Work out the finished part from the listing and answer in its coordinate system (mm). A direction names the side the tool comes from. Coordinates: 2 decimals unless noted, no trailing zeros. Order: outer loops, then holes, each group sorted by start corner. A loop starts at its lowest first (then second) coordinate and runs counter-clockwise, first axis right, second up. Notation, with made-up numbers: (-12.5, -27.75) -> (25.5, -27.75) arc R31 ccw to (25.5, 7.25) -> close; hole circle Ø7 at (47, 4). An arc over 180 degrees is marked (long way). Use one line per item in the form item = value.
Autodesk Fusion 360 part; units mm, degrees
sketch "Sketch1" plane through (0, 0, 0) normal (0, 0, 1) x (1, 0, 0)
  line L0 (27.2658, -132.272) -> (-30, -99.2094)
  line L1 (-30, -99.2094) -> (-30, -33.0822)
  line L2 (-30, -33.0822) -> (27.2658, -0.0196)
  line L3 (27.2658, -0.0196) -> (84.5305, -33.0822)
  line L4 (84.5305, -33.0822) -> (84.5305, -99.2094)
  line L5 (84.5305, -99.2094) -> (27.2658, -132.272)
  line L6 (-8.1812, -86.62) -> (27.2658, -107.0932)
  line L7 (27.2658, -107.0932) -> (62.7117, -86.62)
  line L8 (62.7117, -86.62) -> (62.7117, -45.6716)
  line L9 (62.7117, -45.6716) -> (27.2658, -25.1985)
  line L10 (27.2658, -25.1985) -> (-8.1812, -45.6716)
  line L11 (-8.1812, -45.6716) -> (-8.1812, -86.62)
  line L12 (16.2638, -72.502) -> (16.2638, -47.2612)
  line L13 (38.2046, -59.8516) -> (38.2046, -85.0914)
  line L14 (-30, -33.0822) -> (-30, -99.2094)
  line L15 (-8.1812, -86.62) -> (-8.1812, -45.6716)
  line L16 (-8.1812, -45.6716) -> (27.2658, -25.2594)
  line L17 (27.2658, -25.2594) -> (62.7117, -45.6716)
  line L18 (62.7117, -45.6716) -> (62.7117, -45.7326)
  line L19 (84.5305, -33.0822) -> (27.2658, -0.0196)
  line L20 (27.2658, -0.0196) -> (-30, -33.0822)
  line L21 (38.2046, -59.8516) -> (38.2046, -85.0914)
  line L22 (13.6721, -99.2419) -> (-8.1812, -86.62)
  line L23 (40.8862, -33.0655) -> (62.7117, -45.7326)
  line L24 (27.2658, -25.2594) -> (62.7117, -45.7326)
  line L25 (-8.1812, -86.62) -> (27.2658, -107.0932)
  line L26 (16.2638, -47.2612) -> (40.8862, -33.0655)
  line L27 (27.2658, -25.2594) -> (-8.1812, -45.6716)
  line L28 (-8.1812, -86.62) -> (-8.1812, -45.6716)
  line L29 (-8.1812, -86.62) -> (16.3868, -72.44)
  line L30 (16.3868, -72.44) -> (16.2638, -47.2612)
  line L31 (16.2638, -47.2612) -> (40.8862, -33.0655)
  line L32 (38.2046, -85.0914) -> (13.6721, -99.2419)
  line L33 (13.6721, -99.2419) -> (27.2658, -107.0932)
  line L34 (62.7117, -86.62) -> (62.7117, -45.7326)
  line L35 (27.2658, -107.0932) -> (62.7117, -86.62)
  line L36 (38.2046, -85.0914) -> (38.2046, -59.8516)
  line L37 (38.2046, -59.8516) -> (62.7117, -45.7326)
extrude "Extrude1" add sketch "Sketch1" along normal blind 10 contours L0 L1 L2 L3 L4 L5 L14 L19 L20 | L6 L13 L21 L22 L24 L25 L26 L29 L30 L31 L32 L36 L37 makes body 1
sketch "Sketch2" plane through (0, 0, 10) normal (0, 0, 1) x (1, 0, 0)
  line L0 (62.7117, -45.6716) -> (62.7117, -45.7326)
  line L1 (62.7117, -45.7326) -> (62.7117, -86.62)
  line L2 (62.7117, -86.62) -> (27.2658, -107.0932)
  line L3 (27.2658, -107.0932) -> (13.6721, -99.2419)
  line L4 (13.6721, -99.2419) -> (38.2046, -85.0914)
  line L5 (38.2046, -85.0914) -> (38.2046, -59.8516)
  line L6 (38.2046, -59.8516) -> (62.7117, -45.7326)
  line L7 (40.8333, -33.0959) -> (16.2638, -47.2612)
  line L8 (16.2638, -47.2612) -> (16.3868, -72.44)
  line L9 (16.3868, -72.44) -> (-8.1812, -86.62)
  line L10 (-8.1812, -86.62) -> (-8.1812, -45.6716)
  line L11 (-8.1812, -45.6716) -> (27.2658, -25.1985)
  line L12 (84.5305, -33.0822) -> (27.2658, -0.0196)
  line L13 (27.2658, -0.0196) -> (-30, -33.0822)
  line L14 (-30, -33.0822) -> (-30, -99.2094)
  line L15 (-30, -99.2094) -> (27.2658, -132.272)
  line L16 (27.2658, -132.272) -> (84.5305, -99.2094)
  line L17 (84.5305, -99.2094) -> (84.5305, -33.0822)
extrude "Extrude2" add 1 faces at (3.646, -110.2411, 10) along direction (0, 0, 1) blind 7 separate body on bodies 1 makes body 2
sketch "Sketch3" plane through (0, 0, 17) normal (0, 0, 1) x (1, 0, 0)
  line L0 (62.7117, -45.6716) -> (62.7117, -45.7326)
  line L1 (62.7117, -45.7326) -> (62.7117, -86.62)
  line L2 (62.7117, -86.62) -> (27.2658, -107.0932)
  line L3 (27.2658, -107.0932) -> (13.6721, -99.2419)
  line L4 (13.6721, -99.2419) -> (38.2046, -85.0914)
  line L5 (38.2046, -85.0914) -> (38.2046, -59.8516)
  line L6 (38.2046, -59.8516) -> (62.7117, -45.7326)
  line L7 (40.8333, -33.0959) -> (16.2638, -47.2612)
  line L8 (16.2638, -47.2612) -> (16.3868, -72.44)
  line L9 (16.3868, -72.44) -> (-8.1812, -86.62)
  line L10 (-8.1812, -86.62) -> (-8.1812, -45.6716)
  line L11 (-8.1812, -45.6716) -> (27.2658, -25.1985)
  line L12 (84.5305, -33.0822) -> (27.2658, -0.0196)
  line L13 (27.2658, -0.0196) -> (-30, -33.0822)
  line L14 (-30, -33.0822) -> (-30, -99.2094)
  line L15 (-30, -99.2094) -> (27.2658, -132.272)
  line L16 (27.2658, -132.272) -> (84.5305, -99.2094)
  line L17 (84.5305, -99.2094) -> (84.5305, -33.0822)
  line L18 (-30, -33.0822) -> (27.2658, -0.0196)
  line L19 (84.5305, -33.0822) -> (27.2658, -0.0196)
  line L20 (-30, -33.0822) -> (-30, -99.2094)
  line L21 (-30, -99.2094) -> (27.2658, -132.272)
  line L22 (27.2658, -132.272) -> (84.5305, -99.2094)
  line L23 (84.5305, -33.0822) -> (84.5305, -99.2094)
  line L24 (-8.1812, -45.6716) -> (27.2658, -25.1985)
  line L25 (16.2638, -47.2612) -> (40.8333, -33.0959)
  line L26 (16.2638, -47.2612) -> (16.3868, -72.44)
  line L27 (-8.1812, -86.62) -> (16.3868, -72.44)
  line L28 (-8.1812, -86.62) -> (-8.1812, -45.6716)
  line L29 (62.7117, -45.6716) -> (38.2046, -59.8516)
  line L30 (38.2046, -85.0914) -> (13.6721, -99.2419)
  line L31 (27.2658, -107.0932) -> (13.6721, -99.2419)
  line L32 (27.2658, -107.0932) -> (62.7117, -86.62)
  line L33 (62.7117, -86.62) -> (62.7117, -45.6716)
  line L34 (38.2046, -85.0914) -> (38.2046, -59.8516)
  line L35 (27.2658, -25.1985) -> (40.8333, -33.0959)
  point P0 (27.2658, -25.1985)
extrude "Extrude3" add sketch "Sketch3" along normal blind 5 separate body makes body 3
sketch "Sketch4" plane through (0, 0, 22) normal (0, 0, 1) x (1, 0, 0)
  line L0 (62.7117, -86.62) -> (27.2658, -107.0932)
  line L1 (27.2658, -107.0932) -> (13.6721, -99.2419)
  line L2 (13.6721, -99.2419) -> (38.2046, -85.0914)
  line L3 (38.2046, -85.0914) -> (38.2046, -59.8516)
  line L4 (38.2046, -59.8516) -> (62.7117, -45.6716)
  line L5 (62.7117, -45.6716) -> (62.7117, -86.62)
  line L6 (16.3868, -72.44) -> (-8.1812, -86.62)
  line L7 (-8.1812, -86.62) -> (-8.1812, -45.6716)
  line L8 (-8.1812, -45.6716) -> (27.2658, -25.1985)
  line L9 (27.2658, -25.1985) -> (40.8333, -33.0959)
  line L10 (40.8333, -33.0959) -> (16.2638, -47.2612)
  line L11 (16.2638, -47.2612) -> (16.3868, -72.44)
  line L12 (-30, -33.0822) -> (-30, -99.2094)
  line L13 (-30, -99.2094) -> (27.2658, -132.272)
  line L14 (27.2658, -132.272) -> (84.5305, -99.2094)
  line L15 (84.5305, -99.2094) -> (84.5305, -33.0822)
  line L16 (84.5305, -33.0822) -> (27.2658, -0.0196)
  line L17 (27.2658, -0.0196) -> (-30, -33.0822)
hidden bodies 1 2
(1) Straight lines are drawn through the part: line 1 along X through (y, z) = (-68, 17.35); line 2 along Y through (x, z) = (24, 21.7); line 3 along Y through (x, z) = (16.5, 19.2). For each, find the intervals that lie inside material, in ascending order.
Data:
line_1 = -30 to -8.18, 16.37 to 38.2, 62.71 to 84.53
line_2 = -130.39 to -105.21, -93.28 to -42.8, -27.08 to -1.91
line_3 = -126.06 to -100.88, -97.61 to -47.13, -31.42 to -6.24
(2) The mould has two halves that part along X. Classify faces 3 (the flat face through (26, -65, 22)), 4 (the flat face through (9.29, -35.58, 19.46)), 5 (the flat face through (84.53, -67, 19)): released by +X, released by -X, zero draft, split by the parting line, or undercut.
Data:
face_3 = zero draft
face_4 = undercut
face_5 = released by +X
(3) Section D-D on y = -79 is taken. Write down the section's boundary in (x, z), plus the area to 3 significant figures.
Data:
outline = (-30, 17) -> (-8.18, 17) -> (-8.18, 22) -> (-30, 22) -> close; (5.02, 17) -> (38.2, 17) -> (38.2, 22) -> (5.02, 22) -> close; (62.71, 17) -> (84.53, 17) -> (84.53, 22) -> (62.71, 22) -> close
area = 384 mm²
(4) Which of the six approach directions +Z, -Z, +X, -X, +Y, -Y give full straight-line access (tool end or side, diameter ignored) to faces 1 (the flat face through (55.5, -115.97, 19.46)), 2 (the flat face through (4.275, -79.431, 19.465))?
Data:
face_1 = +Z, -Z, +X, -Y
face_2 = +Z, -Z
(5) Section B-B on x = -5 is taken. Write down the section's boundary in (y, z), plus the area to 3 significant figures.
Data:
outline = (-113.64, 17) -> (-84.78, 17) -> (-84.78, 22) -> (-113.64, 22) -> close; (-43.83, 17) -> (-18.65, 17) -> (-18.65, 22) -> (-43.83, 22) -> close
area = 270 mm²
(6) Section A-A on y = -101 is taken. Write down the section's boundary in (x, z).
Data:
outline = (-26.9, 17) -> (16.72, 17) -> (16.72, 22) -> (-26.9, 22) -> close; (37.82, 17) -> (81.43, 17) -> (81.43, 22) -> (37.82, 22) -> close
(7) Section C-C on z = 20.1 is taken. Write down the section's boundary in (x, y), plus the area to 3 significant figures.
Data:
outline = (-30, -99.21) -> (27.27, -132.27) -> (84.53, -99.21) -> (84.53, -33.08) -> (27.27, -0.02) -> (-30, -33.08) -> close; hole (-8.18, -86.62) -> (16.39, -72.44) -> (16.26, -47.26) -> (40.83, -33.1) -> (27.27, -25.2) -> (-8.18, -45.67) -> close; hole (13.67, -99.24) -> (27.27, -107.09) -> (62.71, -86.62) -> (62.71, -45.67) -> (38.2, -59.85) -> (38.2, -85.09) -> close
area = 8,800 mm²
(8) Each of these flat-tipped pins is pushed along its axis until it touches: P1, Ø1, axis at x = 37.5, z = 19, coming from the +Y side; P2, Ø2, axis at y = -114, z = 17.5, coming from the +X side; P3, Ø3, axis at y = -104, z = 19.5, coming from the -X side. Where does it stop, or does it pass through?
Data:
P1 = -5.64
P2 = 60.65
P3 = -24.3
